Geometry: see drawing. Coordinates: mm, zero at the bounding-box minimum. Give positions to 0.01 mm unless a question says otherwise; leave off trailing zeros. Write each loop counter-clockwise with the first axis right and the second up, starting at its lowest first coordinate (ties: lowest second). Pieces come first, ordered by that corner, then holes. Notation, with made-up numbers: (-31, 67) -> (-26, 67) arc R7 ccw to (-26, 74) -> close; hole circle Ø10 at (-27, 80). An arc over 180 degrees is marked (long way). Answer as a JSON object with one key per item and string values. Group by question number.
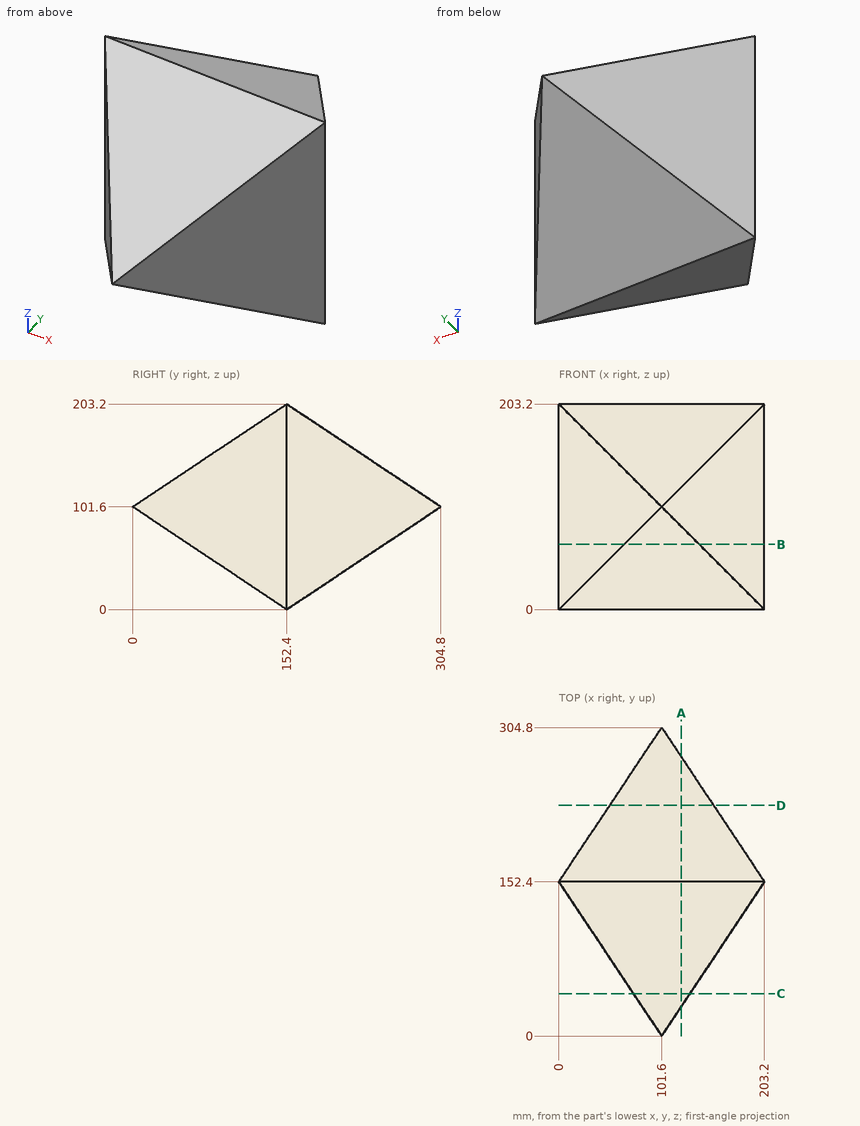
1. Section B-B (z = 64.5). Return the cut outline in (x, y).
2. Section D-D (y = 228). Return the cut outline in (x, z), plus the area to 3 significant figures.
3. Line query: line 1 (Y direction, x = 8, z = 173); line 2 (Z direction, x = 30, y = 170); line 3 (Z direction, x = 148.5, y = 161). Output: solid intervals per line, ascending.
4. Section A-A (x = 121). Return the cut outline in (y, z).
5. Section C-C (y = 42). Return the cut outline in (x, z).
6. Contact query for flat-ended pins moving along their axis: pin 1 Ø1.5 at (x, y) = (62.5, 58) entering from +Z; pin 2 Ø6 at (y, z) = (129, 110.5) entering from +X; pin 3 Ø4 at (x, y) = (110, 46.5) entering from -Z. Output: stop coordinate, or through.
Working result:
{
 "1": {"outline": "(0, 152.4) -> (64.5, 55.65) -> (138.7, 55.65) -> (203.2, 152.4) -> (138.7, 249.15) -> (64.5, 249.15) -> close"},
 "2": {"outline": "(50.4, 50.4) -> (152.8, 50.4) -> (152.8, 152.8) -> (50.4, 152.8) -> close", "area": "10,500 mm^2"},
 "3": {"line 1": "y = 140.4 to 164.4", "line 2": "z = 11.73 to 191.47", "line 3": "z = 5.73 to 197.47"},
 "4": {"outline": "(29.1, 82.2) -> (152.4, 0) -> (275.7, 82.2) -> (275.7, 121) -> (152.4, 203.2) -> (29.1, 121) -> close"},
 "5": {"outline": "(73.6, 73.6) -> (129.6, 73.6) -> (129.6, 129.6) -> (73.6, 129.6) -> close"},
 "6": {"pin 1": "stops at z = 140.77", "pin 2": "stops at x = 189.6", "pin 3": "stops at z = 69.27"}
}
